Work out the finished part from the listing and answer in its coordinate system (mm). Face numbers are marked on the shaded views. A direction names the side the tool comes from. Round coordinates to 2 decimals unless told otherwise and drop trailing zeros. Write each loop counter-clockwise with the first axis right and the second up, starting at its lowest first coordinate (ties: lowest second). Pieces come first, ordered by that corner, then holes.
1. Determine the mould class of the marked faces 1, 2 and 3 for opening direction Z: pulls with the +Z half, pulls with the -Z half, needs draft (parallel to the pull), parting line crosses it, or undercut.
2. Find section D-D (z = 11.5). Write down the section's boundary in (x, y), and give its area (3 significant figures).
3. Flat-ended cylindrical pins translate along their axes: pin 1 Ø5 at (y, z) = (-1.5, 12) entering from -X; pin 2 Ø5 at (y, z) = (-4, 8.5) entering from -X; pin 3 Ø4 at (x, z) = (1, 9.5) entering from -Y. Find the tip coordinate at first contact, or state that the pin passes through.
4. Straight lines are drawn through the part: probe 1 along Z at (x, y) = (4.5, 0.5); probe 2 along X at (y, z) = (0.5, 11.5); probe 3 along X at (y, z) = (0.75, 9.5). For each, find the intervals that lie inside material, in ascending order.
5. A tool of negligible diameter and unlimited length cuts with its end or side. For the marked faces 4, 5 and 6, from which of +Z, -Z, +X, -X, +Y, -Y can it reach the whole face along a straight path? Write none if from no direction.
6. Find section C-C (z = 2). Write down the section's boundary in (x, y).
7. Find section A-A (x = 0). Write down the section's boundary in (y, z).
8. Find section B-B (z = 10). Write down the section's boundary in (x, y), and give its area (3 significant figures).
```python
from build123d import *

# Parameters (mm, degrees)
SKETCH_1_R          = 7.9
EXTRUDE_1_DEPTH     = 5.3
SKETCH_2_W          = 3.6
SKETCH_2_H          = 6
EXTRUDE_2_DEPTH     = 9.7
CUT_EXTRUDE_START   = -3.6
CUT_EXTRUDE_1_DEPTH = 3.6
CHAMFER_1_SIZE      = 1
SKETCH_4_R          = 1.5
EXTRUDE_3_DEPTH     = 2


# Read off the part's stored shape, not the designer's step: 切除-拉伸1
with BuildPart() as part:
    # 草图1 → 凸台-拉伸1 (new body)
    with BuildSketch(Plane.XY):
        Circle(SKETCH_1_R)
    extrude(amount=EXTRUDE_1_DEPTH)

    # 草图2 → 凸台-拉伸2 (add)
    with BuildSketch(Plane.XY.offset(5.3)):
        Rectangle(SKETCH_2_W, SKETCH_2_H)
    extrude(amount=EXTRUDE_2_DEPTH)

    # 切除-拉伸1 outline → 切除-拉伸1 (cut)
    with BuildSketch(Plane.ZY.offset(1.8).offset(CUT_EXTRUDE_START)):
        with BuildLine():
            Line((15, 3), (12, 3))
            ThreePointArc((12, 3), (14.121320344, 2.121320344), (15, 0))
            Line((15, 0), (15, 3))
        make_face()
        with BuildLine():
            Line((15, -3), (15, 0))
            ThreePointArc((15, 0), (14.121320344, -2.121320344), (12, -3))
            Line((12, -3), (15, -3))
        make_face()
    extrude(amount=CUT_EXTRUDE_1_DEPTH, mode=Mode.SUBTRACT)

    # 倒角1
    chamfer_1_edges = [part.edges().sort_by_distance(p)[0] for p in [
        (-7.9, 0, 0),
    ]]
    chamfer(chamfer_1_edges, length=CHAMFER_1_SIZE)

    # 草图4 → 凸台-拉伸3 (add)
    with BuildSketch(Plane.ZY.offset(1.8)):
        with Locations(Location((12, 0, 0), (0, 0, 180))):
            Circle(SKETCH_4_R)
    extrude_3 = extrude(amount=EXTRUDE_3_DEPTH)

    # 镜向1: 凸台-拉伸3 across plane
    add(extrude_3.mirror(Plane(origin=(0, 0, 0), x_dir=(0, 0, 1), z_dir=(1, 0, 0))))


solid = part.part
```
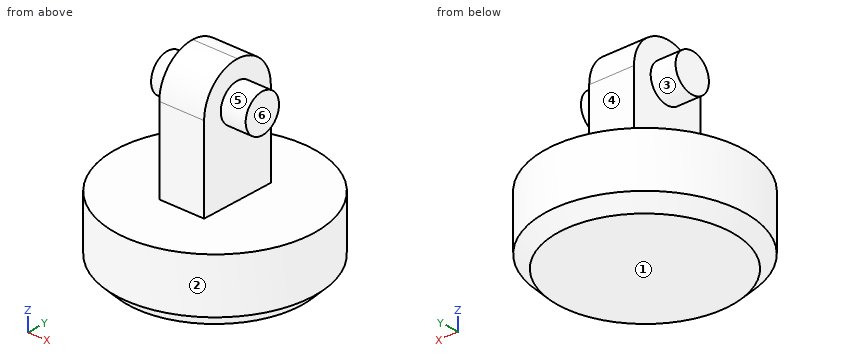
Worked answers:
1. face 1: pulls with the -Z half
1. face 2: needs draft
1. face 3: undercut
2. outline: (-3.8, -1.41) - (-1.8, -1.41) - (-1.8, -3) - (1.8, -3) - (1.8, -1.41) - (3.8, -1.41) - (3.8, 1.41) - (1.8, 1.41) - (1.8, 3) - (-1.8, 3) - (-1.8, 1.41) - (-3.8, 1.41) - close
2. area: 32.9 mm2
3. pin 1: stops at x = -3.8
3. pin 2: stops at x = -1.8
3. pin 3: stops at y = -3
4. probe 1: z = 0 to 5.3
4. probe 2: x = -3.8 to 3.8
4. probe 3: x = -1.8 to 1.8
5. face 4: +Z, +X, -X, +Y
5. face 5: +X
5. face 6: +Z, +X, +Y, -Y
6. outline: circle Ø15.8 at (0, 0)
7. outline: (-7.9, 1) - (-6.9, 0) - (6.9, 0) - (7.9, 1) - (7.9, 5.3) - (3, 5.3) - (3, 12) arc R3 ccw to (-3, 12) - (-3, 5.3) - (-7.9, 5.3) - close
8. outline: (-1.8, -3) - (1.8, -3) - (1.8, 3) - (-1.8, 3) - close
8. area: 21.6 mm2
